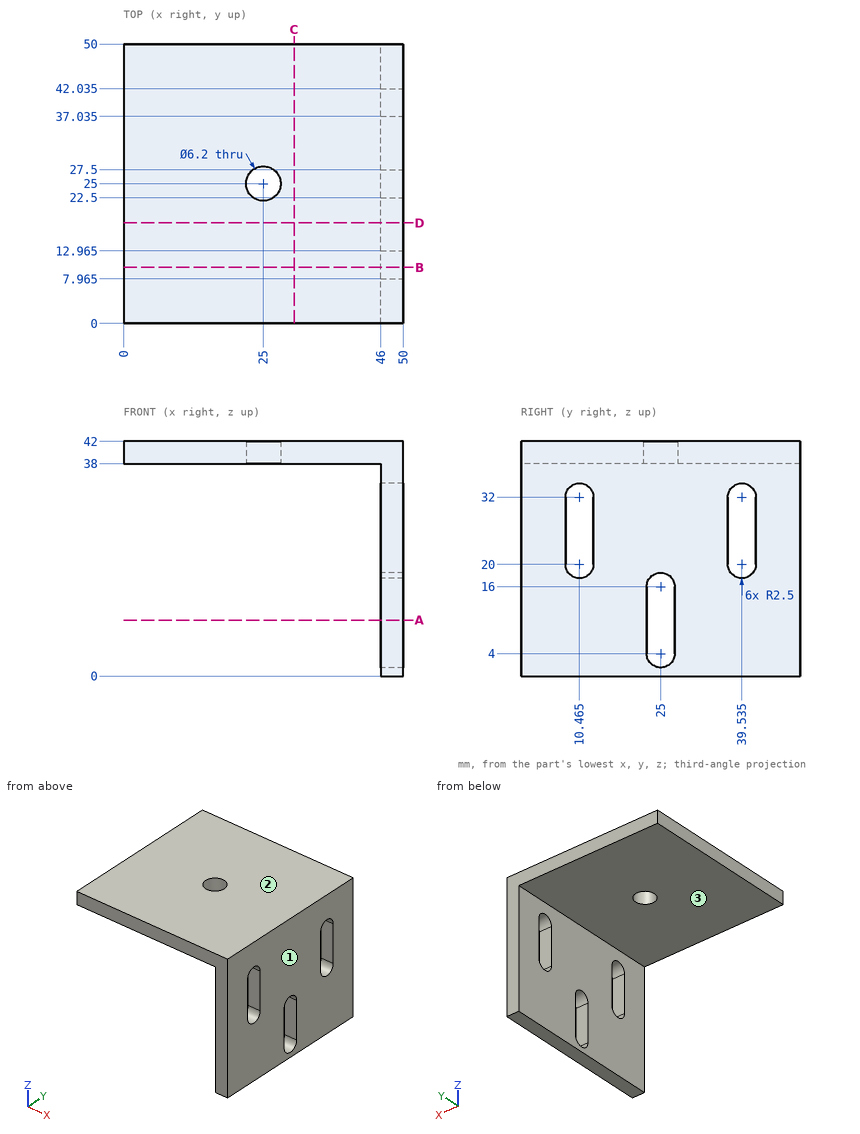
Part print with two shaded views. Sizes in mm from the minimum x, y, z corner. Round coordinates to 2 decimals unless told otherwise and drop trailing zeros. Loops run counter-clockwise (first coordinate to the right, second up) from the corner with the lowest first, then second, coordinate; pieces in that order, holes last. Notation, with made-up numbers: M 60.5,44.5 L 112.5,44.5 A6 ccw 112.5,55.5 Z; hole C -4.5,33 d10. An arc over 180 degrees is marked long. Return JSON: item names as keys, results as strings. Group by question number.
(1) Mould opens along Z. For the marked faces 1, 2 and 3 say: +Z half, -Z half, draft (parallel to the pull), parting line (faces both ways), or undercut.
(2) Drop flat-ended pins along their axis: P1, Ø3.5, axis at x = 25, y = 25, coming from the -Z side; P2, Ø10, axis at x = 35, y = 14, coming from the -Z side; P3, Ø6, axis at y = 25.5, z = 9, coming from the -X side. Give the stop position or say it passes through.
(3) Saw through at C-C, the plane x = 30.5. List the corners of the cut face in (y, z).
(4) Saw through at B-B, the plane y = 10. List the corners of the cut face in (x, z).
(5) Wall check: probe 1 along Y at (x, z) = (25, 39.4); probe 2 along Z at (x, y) = (25.5, 31.5); probe 3 along X at (y, z) = (44, 29). Give the ranges that are in metal, low to high. Write a range as [from, to].
(6) Saw through at D-D, the plane y = 18. List the corners of the cut face in (x, z).
(7) Saw through at A-A, the plane z = 10. List the corners of the cut face in (x, y).
Answer list:
{
 "1": {"face 1": "draft", "face 2": "+Z half", "face 3": "-Z half"},
 "2": {"P1": "through", "P2": "z = 38", "P3": "x = 46"},
 "3": {"outline": "M 0,38 L 50,38 L 50,42 L 0,42 Z"},
 "4": {"outline": "M 0,38 L 46,38 L 46,34.46 L 50,34.46 L 50,42 L 0,42 Z; M 46,0 L 50,0 L 50,17.54 L 46,17.54 Z"},
 "5": {"probe 1": "[0, 21.9], [28.1, 50]", "probe 2": "[38, 42]", "probe 3": "[46, 50]"},
 "6": {"outline": "M 0,38 L 46,38 L 46,0 L 50,0 L 50,42 L 0,42 Z"},
 "7": {"outline": "M 46,0 L 50,0 L 50,22.5 L 46,22.5 Z; M 46,27.5 L 50,27.5 L 50,50 L 46,50 Z"}
}
